Input: part model. Units: mm. Frame: model coordinates. Face numbers are marked on the shaded views. Coordinates: 2 decimals unless noted, no trailing zeros. Write each loop counter-clockwise with the first axis right and the second up, starting at its lowest first coordinate (ties: lowest second). Pieces come first, ordered by that corner, then holes.
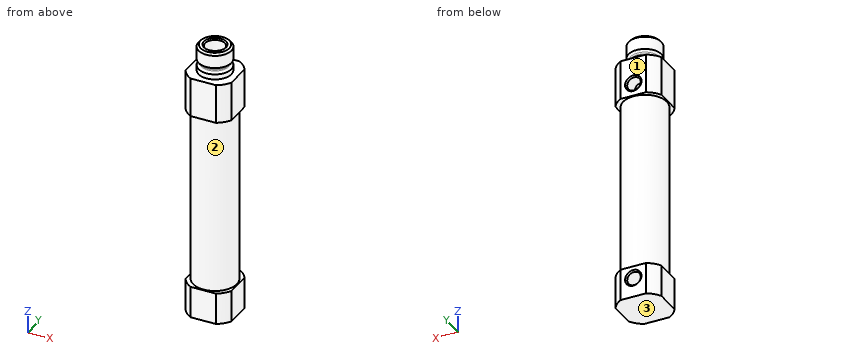
Autodesk Inventor part; units mm, degrees
ref_plane "ANBAU_XY" through (0, 0, 0) normal (0, 0, 1) x (1, 0, 0)
ref_plane "ANBAU_YZ" through (0, 0, 0) normal (1, 0, 0) x (0, 1, 0)
ref_plane "ANBAU_ZX" through (0, 0, 0) normal (0, 1, 0) x (0, 0, 1)
sketch "Sketch_12" plane through (0, 0, 0) normal (1, 0, 0) x (0, 1, 0)
  line L0 (0, -75.85) -> (0, 0)
  line L1 (0, 0) -> (8, 0)
  line L2 (8, 0) -> (8, -11.95)
  line L3 (8, -11.95) -> (6.65, -11.95)
  line L4 (6.65, -11.95) -> (6.65, -66.2)
  line L5 (6.65, -66.2) -> (8, -66.2)
  line L6 (8, -66.2) -> (8, -75.85)
  line L7 (8, -75.85) -> (0, -75.85)
  line L8 (0, -75.85) -> (0, 0)
revolve "Revolution1" add sketch "Sketch_12" angle 360 about axis through (0, 0, -75.85) along (0, 0, -1)
sketch "Sketch_3" plane through (0, 0, 0) normal (1, 0, 0) x (0, 1, 0)
  line L0 (0, 0) -> (0, 8.1)
  line L1 (0, 8.1) -> (4.3865, 8.1)
  line L2 (4.3865, 8.1) -> (5, 7.4865)
  line L3 (5, 7.4865) -> (5, 3.6135)
  line L4 (5, 3.6135) -> (4.3757, 2.9892)
  arc A0 (4.3757, 2.9892) -> (4.2, 2.565) centre (4.8, 2.565) ccw
  line L5 (4.2, 2.565) -> (4.2, 2.2)
  arc A1 (4.2, 2.2) -> (4.8, 1.6) centre (4.8, 2.2) ccw
  line L6 (4.8, 1.6) -> (5, 1.6)
  line L7 (5, 1.6) -> (5, 0)
  line L8 (5, 0) -> (0, 0)
  line L9 (0, 0) -> (0, 8.1)
revolve "Revolution2" add sketch "Sketch_3" angle 360 about axis through (0, 0, 0) along (0, 0, -1)
thread "Thread1"
sketch "Sketch_7" plane through (0, 0, 0) normal (0, 0, 1) x (1, 0, 0)
  line L0 (-14, 14) -> (-14, -14)
  line L1 (-14, -14) -> (14, -14)
  line L2 (14, -14) -> (14, 14)
  line L3 (14, 14) -> (-14, 14)
  line L4 (-7, 7) -> (-7, -7)
  line L5 (-7, -7) -> (7, -7)
  line L6 (7, -7) -> (7, 7)
  line L7 (7, 7) -> (-7, 7)
extrude "Extrusion1" cut sketch "Sketch_7" against normal blind 75.85
sketch "Sketch4" plane through (-3.873, 7, -11.95) normal (0, 1, 0) x (1, 0, 0)
  point P0 (3.873, -3.95)
hole "Hole1" at (0, 7, -8) direction (0, -1, 0) diameter 4.134 depth 7 countersink diameter 5 countersink angle 90
sketch "Sketch5" plane through (-3.873, 7, -66.2) normal (0, 1, 0) x (1, 0, 0)
  point P0 (3.873, 3.65)
hole "Hole2" at (0, 7, -69.85) direction (0, -1, 0) diameter 4.134 depth 11 tip angle 120 countersink diameter 5 countersink angle 90
sketch "Sketch_10" plane through (0, 0, 0) normal (1, 0, 0) x (0, 1, 0)
  line L0 (0, -57) -> (0, 8.1)
  line L1 (0, 8.1) -> (3.4, 8.1)
  line L2 (3.4, 8.1) -> (3, 7.7)
  line L3 (3, 7.7) -> (3, -17)
  line L4 (3, -17) -> (6, -17)
  line L5 (6, -17) -> (6, -57)
  line L6 (6, -57) -> (0, -57)
  line L7 (0, -57) -> (0, 8.1)
revolve "Revolution3" cut sketch "Sketch_10" angle 360 about axis through (0, 0, -57) along (0, 0, -1)
ref_plane "ANBAU_XY" through (0, 0, 0) normal (0, 0, 1) x (1, 0, 0)
ref_plane "ANBAU_YZ" through (0, 0, 0) normal (1, 0, 0) x (0, 1, 0)
ref_plane "ANBAU_ZX" through (0, 0, 0) normal (0, 1, 0) x (0, 0, 1)
ref_plane "FDT_FRONT_XY" through (0, 0, 0) normal (0, 0, -1) x (-1, 0, 0)
ref_plane "FDT_FRONT_YZ" through (0, 0, 0) normal (-1, 0, 0) x (0, 1, 0)
ref_plane "FDT_FRONT_ZX" through (0, 0, 0) normal (0, 1, 0) x (0, 0, -1)
ref_plane "FDT_QSFRONT_XY" through (0, 7, -8) normal (0, 1, 0) x (1, 0, 0)
ref_plane "FDT_QSFRONT_YZ" through (0, 7, -8) normal (1, 0, 0) x (0, 0, -1)
ref_plane "FDT_QSFRONT_ZX" through (0, 7, -8) normal (0, 0, -1) x (0, 1, 0)
ref_plane "FDT_QSREAR_XY" through (0, 7, -69.85) normal (0, 1, 0) x (1, 0, 0)
ref_plane "FDT_QSREAR_YZ" through (0, 7, -69.85) normal (1, 0, 0) x (0, 0, -1)
ref_plane "FDT_QSREAR_ZX" through (0, 7, -69.85) normal (0, 0, -1) x (0, 1, 0)
ref_plane "FDT_REAR_XY" through (0, 0, -75.85) normal (0, 0, 1) x (-1, 0, 0)
ref_plane "FDT_REAR_YZ" through (0, 0, -75.85) normal (-1, 0, 0) x (0, -1, 0)
ref_plane "FDT_REAR_ZX" through (0, 0, -75.85) normal (0, -1, 0) x (0, 0, 1)
ref_plane "FDT_SMBR1_XY" through (0, 0, -21.45) normal (0, 0, 1) x (1, 0, 0)
ref_plane "FDT_SMBR1_YZ" through (0, 0, -21.45) normal (1, 0, 0) x (0, 1, 0)
ref_plane "FDT_SMBR1_ZX" through (0, 0, -21.45) normal (0, 1, 0) x (0, 0, 1)
ref_plane "FDT_SMBR2_XY" through (0, 0, -56.7) normal (0, 0, 1) x (1, 0, 0)
ref_plane "FDT_SMBR2_YZ" through (0, 0, -56.7) normal (1, 0, 0) x (0, 1, 0)
ref_plane "FDT_SMBR2_ZX" through (0, 0, -56.7) normal (0, 1, 0) x (0, 0, 1)
ref_plane "to_nut_XY" through (0, 0, 3.6) normal (0, 0, 1) x (1, 0, 0)
ref_plane "to_nut_YZ" through (0, 0, 3.6) normal (1, 0, 0) x (0, 1, 0)
ref_plane "to_nut_ZX" through (0, 0, 3.6) normal (0, 1, 0) x (0, 0, 1)
ref_plane "to_piston_XY" through (0, 0, -57) normal (0, 0, 1) x (1, 0, 0)
ref_plane "to_piston_YZ" through (0, 0, -57) normal (1, 0, 0) x (0, 1, 0)
ref_plane "to_piston_ZX" through (0, 0, -57) normal (0, 1, 0) x (0, 0, 1)
sketch "Szkic7" plane through (0, 0, -17) normal (0, 0, -1) x (-1, 0, 0)
  circle A0 centre (0, 2.745) radius 0.5831
  point P0 (0, 0)
extrude "Wyciągnięcie proste2" cut sketch "Szkic7" against normal blind 9.5
sketch "Szkic8" plane through (0, 0, -57) normal (0, 0, 1) x (1, 0, 0)
  circle A0 centre (0, -1.5) radius 1.5
  point P0 (0, 0)
extrude "Wyciągnięcie proste3" cut sketch "Szkic8" against normal blind 12.5
properties part number "Korpus"
Item 1: Material intervals for line 1 (Z direction, x = -4.5, y = 2.25); line 2 (X direction, y = 0.25, z = -69.85); line 3 (Z direction, x = 3.5, y = 3), sorted ascending.
Item 2: Pull-direction query (Z, two-part tool) for the marked faces 1, 2 and 3; classes: released by +Z, released by -Z, zero draft, split by the parting line, or undercut.
Item 3: Section query B-B, the plane z = -41. Return loops of the section in (x, y).
Item 4: Pin query (flat end, axial travel): pin 1 Ø2 at (y, z) = (-5, -21.5) entering from +X; pin 2 Ø3 at (x, y) = (0.5, -1) entering from +Z; pin 3 Ø6 at (x, z) = (0.5, -16) entering from -Y. Return the tip coordinate at first contact, or that it passes through.
Item 5: Section query A-A, the plane z = -8. Return loops of the section in (x, y).
The answers:
1. line 1: z = -75.85 to -57, -17 to 0
1. line 2: x = -7 to -2.07, 2.07 to 7
1. line 3: z = -75.85 to -57, -17 to 1.63, 3.22 to 7.88
2. face 1: zero draft
2. face 2: undercut
2. face 3: released by -Z
3. outline: circle Ø13.3 at (0, 0); hole circle Ø12 at (0, 0)
4. pin 1: stops at x = 5.31
4. pin 2: stops at z = -57
4. pin 3: stops at y = -6.65
5. outline: (-7, -3.87) arc R8 ccw to (-3.87, -7) - (3.87, -7) arc R8 ccw to (7, -3.87) - (7, 3.87) arc R8 ccw to (3.87, 7) - (2.5, 7) - (2.07, 6.57) - (2.07, 2.17) arc R3 cw (long way) to (-2.07, 2.17) - (-2.07, 6.57) - (-2.5, 7) - (-3.87, 7) arc R8 ccw to (-7, 3.87) - close
